from build123d import *

# Parameters (mm, degrees)
F0_W     = 19
F0_H     = 10
F0_R     = 3.5
F1_DEPTH = 10
F2_W     = 28.999740434
F2_H     = 5
F3_DEPTH = 20
F4_R     = 1.5
F4_R_2   = 1.5122777257
F5_DEPTH = 25
F6_SIZE  = 5
F7_R     = 1
F8_R     = 1
F9_R     = 2


with BuildPart() as f1:
    # F0 (on Front) → F1 (new body)
    with BuildSketch(Plane.XZ):
        with Locations((9.5, 5)):
            Rectangle(F0_W, F0_H)
        with Locations((4.5, 4.5)):
            Circle(F0_R, mode=Mode.SUBTRACT)
        with Locations((14.5, 4.5)):
            Circle(F0_R, mode=Mode.SUBTRACT)
        Polygon((-4.999931565, 9.9738400144), (0, 10), (19, 10), (24, 10), (23.9767846348, 14.9999461044), (-5.0226432074, 14.8652981916), align=None)
    extrude(amount=F1_DEPTH)

    # F2 (on face) → F3 (join)
    with BuildSketch(Plane(origin=(-0.0691282, 0, 14.8882979715), x_dir=(0.9999892209, 0, 0.004643073), z_dir=(-0.004643073, 0, 0.9999892209))):
        with Locations((9.5463018144, -2.5)):
            Rectangle(F2_W, F2_H)
    extrude(amount=F3_DEPTH)

    # F4 (on face) → F5 (join)
    with BuildSketch(Plane.XZ.offset(5)):
        with Locations((4.6989777146, 21)):
            Circle(F4_R)
        with Locations((15.1989777146, 21)):
            Circle(F4_R_2)
    extrude(amount=-F5_DEPTH)

    # F6
    f6_edges = [f1.edges().sort_by_distance(p)[0] for p in [
        (-5.115505, -2.5, 34.865083),
        (23.883923, -2.5, 34.999731),
    ]]
    chamfer(f6_edges, length=F6_SIZE)

    # F7
    f7_edges = [f1.edges().sort_by_distance(p)[0] for p in [
        (3.198978, 20, 21),
        (13.6867, 20, 21),
    ]]
    fillet(f7_edges, radius=F7_R)

    # F8
    f8_edges = [f1.edges().sort_by_distance(p)[0] for p in [
        (19, -5, 0),
        (0, -5, 0),
    ]]
    fillet(f8_edges, radius=F8_R)

    # F9
    f9_edges = [f1.edges().sort_by_distance(p)[0] for p in [
        (19, -5, 10),
        (0, -5, 10),
    ]]
    fillet(f9_edges, radius=F9_R)


solid = f1.part
Read the model definition and answer for the solid it produces. Units are mm, in the model's axes. A direction names the side the tool comes from. Coordinates: 2 decimals unless noted, no trailing zeros. Loops run counter-clockwise (first coordinate to the right, second up) from the corner with the lowest first, then second, coordinate; pieces in that order, holes last. Notation, with made-up numbers: (71, 82.25) -> (77, 82.25) arc R31 cw to (77, 115.25) -> close; hole circle Ø11 at (26.5, 72.25). An arc over 180 degrees is marked (long way). Answer in a Markdown table with one row per item.
Item 1: For faces 1 (the flat face through (9, -5, 25)), 2 (the flat face through (19, -5, 4)), 3 (the flat face through (0, -5, 4)), determine the directions among +Z, -Z, +X, -X, +Y, -Y from which every point of the face is accessible in a straight line to the end or side of a thin tool.
Returned:
| item | result |
|---|---|
| face 1 | +Z, +X, -X, -Y |
| face 2 | -Z, +X, +Y, -Y |
| face 3 | -Z, -X, +Y, -Y |
Item 2: A cutting plane is placed at D-D on x = 20. Determine the outline of the cut face in (y, z), plus the area to 3 significant figures.
Returned:
| item | result |
|---|---|
| outline | (-10, 9.73) -> (0, 9.73) -> (0, 33.87) -> (-5, 33.87) -> (-5, 14.98) -> (-10, 14.98) -> close |
| area | 147 mm^2 |
Item 3: For a pull along X with two mould halves and no side action, classify faces 4 (the cylindrical face through (4.504, 9.367, 22.487)), 5 (the flat face through (5, 20, 21)), 6 (the flat face through (21.431, -2.535, 32.453)) as released by +X, released by -X, zero draft, split by the parting line, or undercut.
Returned:
| item | result |
|---|---|
| face 4 | undercut |
| face 5 | zero draft |
| face 6 | released by +X |
Item 4: A cutting plane is placed at B-B on y = -7.5. Determine the outline of the cut face in (x, z).
Returned:
| item | result |
|---|---|
| outline | (-5.02, 14.87) -> (-5, 9.97) -> (-2.01, 9.99) arc R2 cw to (0, 7.99) -> (0, 1) arc R1 ccw to (1, 0) -> (18, 0) arc R1 ccw to (19, 1) -> (19, 8) arc R2 cw to (21, 10) -> (24, 10) -> (23.98, 15) -> close; hole circle Ø7 at (4.5, 4.5); hole circle Ø7 at (14.5, 4.5) |
Item 5: Straight lines are drawn through the part: line 1 along Y through (x, z) = (9.75, 22.5); line 2 along Z through (x, y) = (4.5, -6); line 3 along X through (y, z) = (8.5, 20.5). For each, find the intervals that lie inside material, in ascending order. Write a range as [from, to].
Returned:
| item | result |
|---|---|
| line 1 | y = [-5, 0] |
| line 2 | z = [0, 1], [8, 14.91] |
| line 3 | x = [3.28, 6.11], [13.77, 16.63] |
Item 6: Each of these flat-tipped pins is pushed along its axis until it touches: P1, Ø4, axis at y = 1.5, z = 7.5, coming from the +X side; P2, Ø2, axis at y = -3, z = 5, coming from the +X side; P3, Ø7.5, axis at y = -7, z = 5.5, coming from the -X side. Where does it stop, or does it pass through?
Returned:
| item | result |
|---|---|
| P1 | stops at x = 19.18 |
| P2 | stops at x = 19 |
| P3 | stops at x = -0.45 |
Item 7: A cutting plane is placed at C-C on x = 7.25. Determine the outline of the cut face in (y, z).
Returned:
| item | result |
|---|---|
| outline | (-10, 0) -> (0, 0) -> (0, 2.33) -> (-10, 2.33) -> close; (-10, 6.67) -> (0, 6.67) -> (0, 34.92) -> (-5, 34.92) -> (-5, 14.92) -> (-10, 14.92) -> close |
Item 8: A cutting plane is placed at A-A on z = 4.5. Determine the outline of the cut face in (x, y), plus the area to 3 significant figures.
Returned:
| item | result |
|---|---|
| outline | (0, -10) -> (1, -10) -> (1, 0) -> (0, 0) -> close; (8, -10) -> (11, -10) -> (11, 0) -> (8, 0) -> close; (18, -10) -> (19, -10) -> (19, 0) -> (18, 0) -> close |
| area | 50.0 mm^2 |
